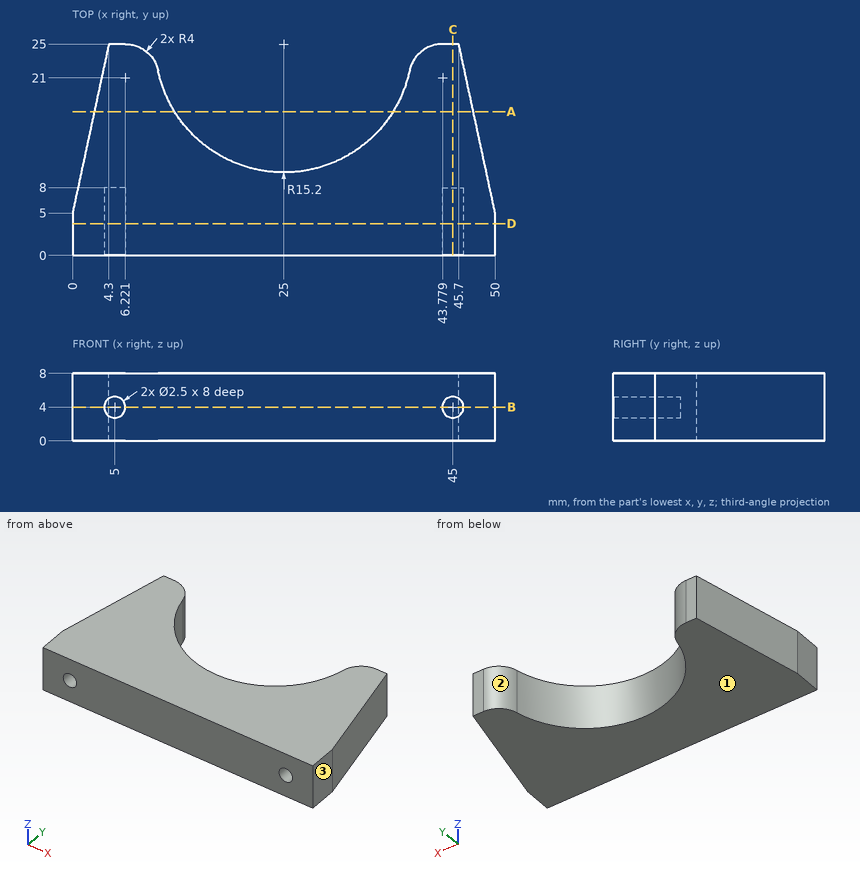
Part print with two shaded views. Sizes in mm from the minimum x, y, z corner. Round coordinates to 2 decimals unless told otherwise and drop trailing zeros. Order: outer loops, then holes, each group sorted by start corner. A loop starts at its lowest first (then second) coordinate and runs counter-clockwise, first axis right, second up.
(1) Band-saw the part on C-C (x = 45). List the corners of the cut face in (y, z).
(2) Band-saw the part on B-B (z = 4). List the corners of the cut face in (x, y), then the cut area to 3 significant figures.
(3) Band-saw the part on D-D (y = 3.75). List the corners of the cut face in (x, z).
(4) Band-saw the part on A-A (y = 17). List the corners of the cut face in (x, z).
(5) Drill centre lines: line 1 (X direction, y = 4, z = 4); line 2 (Z direction, x = 45, y = 4); line 3 (X direction, y = 12, z = 6) (1 decimal). Where is each one in solid material? Low to high.
(6) Pin check, flat tips, straight feed: pin 1 (3 mm diameter, centred on x = 41, z = 7, fed in from +Y); pin 2 (1 mm diameter, centred on y = 10, z = 1.5, fed in from -X); pin 3 (1.5 mm diameter, centred on y = 14.5, z = 4.5, fed in from -X). Stop position of each tip, or through.
(7) Pull direction X, two halves, no side cores. Call the marked faces 1, 2 and 3: released by +X, released by -X, zero draft, split by the parting line, or undercut.
Verdict:
1. outline: (0, 0) - (25, 0) - (25, 8) - (0, 8) - (0, 5.25) - (8, 5.25) - (8, 2.75) - (0, 2.75) - close
2. outline: (0, 0) - (3.75, 0) - (3.75, 8) - (6.25, 8) - (6.25, 0) - (43.75, 0) - (43.75, 8) - (46.25, 8) - (46.25, 0) - (50, 0) - (50, 5) - (45.7, 25) - (43.78, 25) arc R4 ccw to (39.87, 21.83) arc R15.2 cw to (10.13, 21.83) arc R4 ccw to (6.22, 25) - (4.3, 25) - (0, 5) - close
2. area: 756 mm2
3. outline: (0, 0) - (50, 0) - (50, 8) - (0, 8) - close; hole circle Ø2.5 at (5, 4); hole circle Ø2.5 at (45, 4)
4. outline: (2.58, 0) - (12.08, 0) - (12.08, 8) - (2.58, 8) - close; (37.92, 0) - (47.42, 0) - (47.42, 8) - (37.92, 8) - close
5. line 1: x = 0 to 3.75, 6.25 to 43.75, 46.25 to 50
5. line 2: z = 0 to 2.75, 5.25 to 8
5. line 3: x = 1.5 to 17.1, 32.9 to 48.5
6. pin 1: stops at y = 24.79
6. pin 2: stops at x = 0.97
6. pin 3: stops at x = 1.88
7. face 1: zero draft
7. face 2: undercut
7. face 3: released by +X
